```python
from build123d import *

# Parameters (mm, degrees)
SKETCH1_W            = 920.75
SKETCH1_H            = 416.56
BOSS_EXTRUDE1_DEPTH  = 6.35
SKETCH2_W            = 920.75
SKETCH2_H            = 25.4
BOSS_EXTRUDE2_DEPTH  = 6.35
SKETCH3_W            = 57.15
SKETCH3_H            = 13.97
TAB_HOLES_DEPTH      = 517.442419854
SKETCH4_W            = 25.4
SKETCH4_H            = 50.8
SKETCH4_R            = 5.3578125
TABS_DEPTH           = 6.35
FILLET1_R            = 3.175
FILLET2_R            = 3.175
FILLET2_OF_MIRROR2_R = 3.175
MIRROR4_START        = -6.35
MIRROR4_DEPTH        = 12.7
MIRROR4_2_OUTLINE_R  = 5.3578125
MIRROR4_2_DEPTH      = 12.7
FILLET3_R            = 3.175


# Read off the part's stored shape, not the designer's step: Mirror4
with BuildPart() as part:
    # Sketch1 → Boss-Extrude1 (new, symmetric)
    with BuildSketch(Plane.XY):
        Rectangle(SKETCH1_W, SKETCH1_H)
    extrude(amount=BOSS_EXTRUDE1_DEPTH, both=True)

    # Sketch2 → Boss-Extrude2 (add, symmetric)
    with BuildSketch(Plane.XY):
        with Locations((0, 220.98)):
            Rectangle(SKETCH2_W, SKETCH2_H)
        with Locations((0, -220.98)):
            Rectangle(SKETCH2_W, SKETCH2_H)
    extrude(amount=BOSS_EXTRUDE2_DEPTH, both=True)

    # Sketch3 → Tab Holes (cut, through all)
    with BuildSketch(Plane.XY.offset(6.35)):
        with Locations((-345.28125, 215.265)):
            Rectangle(SKETCH3_W, SKETCH3_H)
        with Locations((-115.09375, 215.265)):
            Rectangle(SKETCH3_W, SKETCH3_H)
    tab_holes = extrude(amount=-TAB_HOLES_DEPTH, mode=Mode.SUBTRACT)

    # Sketch4 → Tabs (add, symmetric)
    # profile 1 of 2: a face of its own
    with BuildSketch(Plane.XY):
        with Locations((-473.075, 104.14)):
            Rectangle(SKETCH4_W, SKETCH4_H)
        with Locations((-472.28125, 104.14)):
            Circle(SKETCH4_R, mode=Mode.SUBTRACT)
    # profile 2 of 2: a face of its own
    with BuildSketch(Plane.XY):
        with Locations((-473.075, -104.14)):
            Rectangle(SKETCH4_W, SKETCH4_H)
        with Locations((-472.28125, -104.14)):
            Circle(SKETCH4_R, mode=Mode.SUBTRACT)
    extrude(amount=TABS_DEPTH, both=True)

    # Fillet1
    fillet1_edges = [part.edges().sort_by_distance(p)[0] for p in [
        (-460.375, 233.68, 0),
        (-460.375, -233.68, 0),
        (-460.375, 78.74, 0),
        (-460.375, 129.54, 0),
        (-485.775, 129.54, 0),
        (-485.775, 78.74, 0),
        (-460.375, -129.54, 0),
        (-460.375, -78.74, 0),
        (-485.775, -78.74, 0),
        (-485.775, -129.54, 0),
    ]]
    fillet(fillet1_edges, radius=FILLET1_R)

    # Fillet2
    fillet2_edges = [part.edges().sort_by_distance(p)[0] for p in [
        (-373.85625, 208.28, 0),
        (-373.85625, 222.25, 0),
        (-316.70625, 222.25, 0),
        (-316.70625, 208.28, 0),
        (-143.66875, 208.28, 0),
        (-143.66875, 222.25, 0),
        (-86.51875, 222.25, 0),
        (-86.51875, 208.28, 0),
    ]]
    fillet(fillet2_edges, radius=FILLET2_R)

    # Mirror2: Tab Holes across plane
    add(tab_holes.mirror(Plane.ZX), mode=Mode.SUBTRACT)

    # Fillet2 of Mirror2
    fillet2_of_mirror2_edges = [part.edges().sort_by_distance(p)[0] for p in [
        (-373.85625, -208.28, 0),
        (-373.85625, -222.25, 0),
        (-316.70625, -222.25, 0),
        (-316.70625, -208.28, 0),
        (-143.66875, -208.28, 0),
        (-143.66875, -222.25, 0),
        (-86.51875, -222.25, 0),
        (-86.51875, -208.28, 0),
    ]]
    fillet(fillet2_of_mirror2_edges, radius=FILLET2_OF_MIRROR2_R)

    # Mirror4 outline → Mirror4 (cut)
    with BuildSketch(Plane.XY.offset(MIRROR4_START)):
        with BuildLine():
            Line((140.49375, 222.25), (89.69375, 222.25))
            ThreePointArc((89.69375, 222.25), (87.44868597, 221.32006403), (86.51875, 219.075))
            Line((86.51875, 219.075), (86.51875, 211.455))
            ThreePointArc((86.51875, 211.455), (87.44868597, 209.20993597), (89.69375, 208.28))
            Line((89.69375, 208.28), (140.49375, 208.28))
            ThreePointArc((140.49375, 208.28), (142.73881403, 209.20993597), (143.66875, 211.455))
            Line((143.66875, 211.455), (143.66875, 219.075))
            ThreePointArc((143.66875, 219.075), (142.73881403, 221.32006403), (140.49375, 222.25))
        make_face()
        with BuildLine():
            Line((370.68125, 222.25), (319.88125, 222.25))
            ThreePointArc((319.88125, 222.25), (317.63618597, 221.32006403), (316.70625, 219.075))
            Line((316.70625, 219.075), (316.70625, 211.455))
            ThreePointArc((316.70625, 211.455), (317.63618597, 209.20993597), (319.88125, 208.28))
            Line((319.88125, 208.28), (370.68125, 208.28))
            ThreePointArc((370.68125, 208.28), (372.92631403, 209.20993597), (373.85625, 211.455))
            Line((373.85625, 211.455), (373.85625, 219.075))
            ThreePointArc((373.85625, 219.075), (372.92631403, 221.32006403), (370.68125, 222.25))
        make_face()
        with BuildLine():
            ThreePointArc((143.66875, -211.455), (142.73881403, -209.20993597), (140.49375, -208.28))
            Line((140.49375, -208.28), (89.69375, -208.28))
            ThreePointArc((89.69375, -208.28), (87.44868597, -209.20993597), (86.51875, -211.455))
            Line((86.51875, -211.455), (86.51875, -219.075))
            ThreePointArc((86.51875, -219.075), (87.44868597, -221.32006403), (89.69375, -222.25))
            Line((89.69375, -222.25), (140.49375, -222.25))
            ThreePointArc((140.49375, -222.25), (142.73881403, -221.32006403), (143.66875, -219.075))
            Line((143.66875, -219.075), (143.66875, -211.455))
        make_face()
        with BuildLine():
            ThreePointArc((373.85625, -211.455), (372.92631403, -209.20993597), (370.68125, -208.28))
            Line((370.68125, -208.28), (319.88125, -208.28))
            ThreePointArc((319.88125, -208.28), (317.63618597, -209.20993597), (316.70625, -211.455))
            Line((316.70625, -211.455), (316.70625, -219.075))
            ThreePointArc((316.70625, -219.075), (317.63618597, -221.32006403), (319.88125, -222.25))
            Line((319.88125, -222.25), (370.68125, -222.25))
            ThreePointArc((370.68125, -222.25), (372.92631403, -221.32006403), (373.85625, -219.075))
            Line((373.85625, -219.075), (373.85625, -211.455))
        make_face()
    extrude(amount=MIRROR4_DEPTH, mode=Mode.SUBTRACT)

    # Mirror4 2 outline → Mirror4 2 (add)
    # profile 1 of 2: a face of its own
    with BuildSketch(Plane.XY.offset(MIRROR4_START)):
        with BuildLine():
            ThreePointArc((485.775, 126.365), (484.84506403, 128.61006403), (482.6, 129.54))
            Line((482.6, 129.54), (460.375, 129.54))
            Line((460.375, 129.54), (460.375, 78.74))
            Line((460.375, 78.74), (482.6, 78.74))
            ThreePointArc((482.6, 78.74), (484.84506403, 79.66993597), (485.775, 81.915))
            Line((485.775, 81.915), (485.775, 126.365))
        make_face()
        with Locations((472.28125, 104.14)):
            Circle(MIRROR4_2_OUTLINE_R, mode=Mode.SUBTRACT)
    # profile 2 of 2: a face of its own
    with BuildSketch(Plane.XY.offset(MIRROR4_START)):
        with BuildLine():
            Line((482.6, -78.74), (460.375, -78.74))
            Line((460.375, -78.74), (460.375, -129.54))
            Line((460.375, -129.54), (482.6, -129.54))
            ThreePointArc((482.6, -129.54), (484.84506403, -128.61006403), (485.775, -126.365))
            Line((485.775, -126.365), (485.775, -81.915))
            ThreePointArc((485.775, -81.915), (484.84506403, -79.66993597), (482.6, -78.74))
        make_face()
        with Locations((472.28125, -104.14)):
            Circle(MIRROR4_2_OUTLINE_R, mode=Mode.SUBTRACT)
    extrude(amount=MIRROR4_2_DEPTH)

    # Fillet3
    fillet3_edges = [part.edges().sort_by_distance(p)[0] for p in [
        (460.375, 233.68, 0),
        (460.375, -233.68, 0),
        (460.375, 129.54, 0),
        (460.375, 78.74, 0),
        (460.375, -78.74, 0),
        (460.375, -129.54, 0),
    ]]
    fillet(fillet3_edges, radius=FILLET3_R)


solid = part.part
```
Can you work these out from the model? Positions are in its coordinate system, mm. Coordinates: 2 decimals unless noted, no trailing zeros. Loops run counter-clockwise (first coordinate to the right, second up) from the corner with the lowest first, then second, coordinate; pieces in that order, holes last. Notation, with made-up numbers: M -21,-30.75 L -1,-30.75 A25 ccw -1,-12.75 Z; hole C -7,24.25 d3. An arc over 180 degrees is marked long. Put each result on its own line as item: value. Start each with the question number.
(1) Imagine slicing it at A-A on z = 1. Give the number of separate pieces and of enclosed holes in the cut face, and give its area (3 significant figures).
(2) I need wall thicknesses on probe 1 along Y at (x, z) = (93, -5.25); probe 2 along X at (y, z) = (-134, -4.5) (3 decimals); probe 3 along X at (y, z) = (129, 1). Which ranges of each line are inside material? Lowest first, please.
(3) Imagine slicing it at B-B on y = -46. List the corners of the cut face in (x, z) for me (3 decimals).
(4) Will these pins go through, and if not, where does the flat tip stop? pin 1 Ø6 at (y, z) = (-143, -4.5) entering from -X (3 decimals); pin 2 Ø4 at (x, z) = (-474, -2.5) entering from +Y; pin 3 Ø2 at (y, z) = (-18.5, 4.5) entering from +X (3 decimals).
Worked answers:
1. separate pieces: 1
1. enclosed holes: 12
1. area: 429,000 mm2
2. probe 1: y = -233.68 to -222.25, -208.28 to 208.28, 222.25 to 233.68
2. probe 2: x = -460.375 to 460.375
2. probe 3: x = -484.37 to 484.37
3. outline: M -460.375,-6.35 L 460.375,-6.35 L 460.375,6.35 L -460.375,6.35 Z
4. pin 1: stops at x = -460.375
4. pin 2: stops at y = 129.54
4. pin 3: stops at x = 460.375
